For this review, use the dimensioned drawing (mm, ordinates from the lowest corner) and the shaded views. A direction names the side the tool comes from. Round coordinates to 2 decimals unless told otherwise and drop trailing zeros. Write each loop counter-clockwise with the first axis right and the second up, starting at its lowest first coordinate (ties: lowest second). Pieces come first, ordered by that corner, then holes. Notation, with made-up numbers: (-23, -15) - (-7, -15) arc R28 cw to (-7, 19) - close; hole circle Ø1 at (11.25, -30). An arc over 180 degrees is marked (long way). Write each question's results on one line, items separated by ' | '.
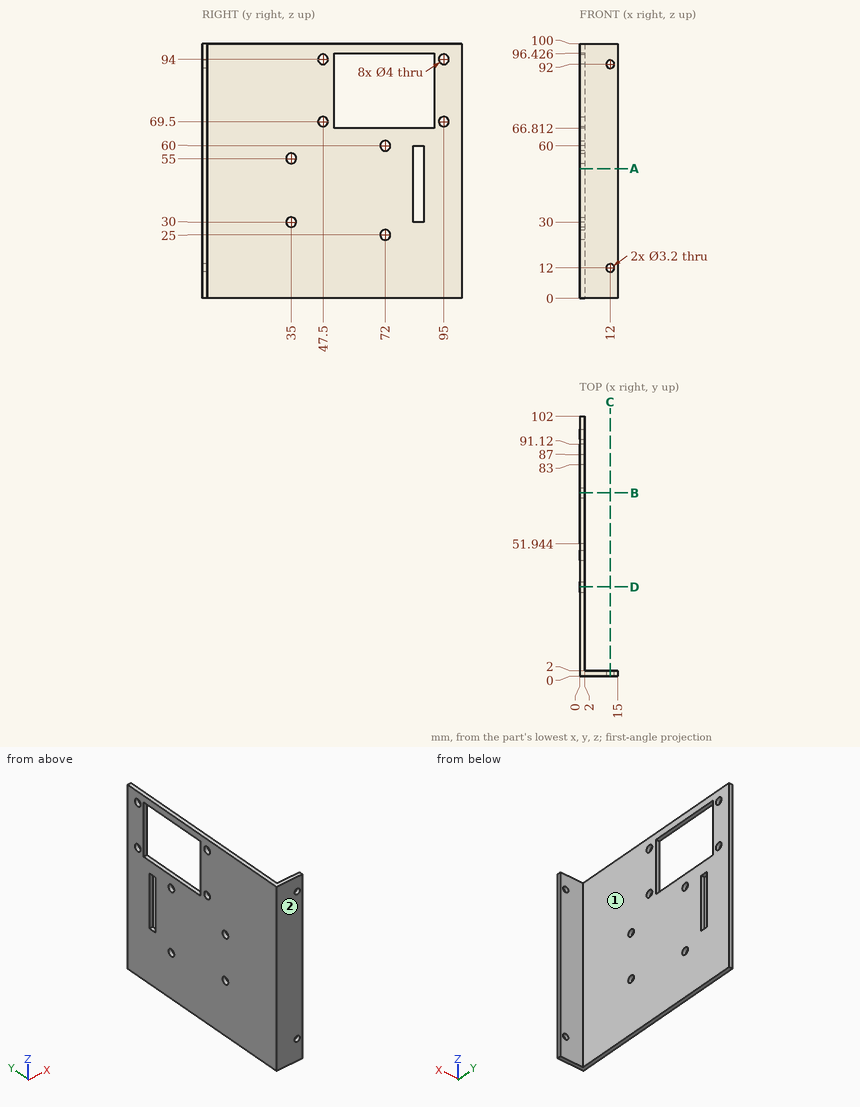
Q1. We need section C-C (x = 12). State the section outline as (y, z) points, plus the area to 3 significant figures.
Evaluation:
outline: (0, 0) - (2, 0) - (2, 10.4) - (0, 10.4) - close; (0, 13.6) - (2, 13.6) - (2, 90.4) - (0, 90.4) - close; (0, 93.6) - (2, 93.6) - (2, 100) - (0, 100) - close | area: 187 mm^2
Q2. We need section A-A (z = 51). State the section outline as (x, y) points.
Evaluation:
outline: (0, 0) - (15, 0) - (15, 2) - (2, 2) - (2, 83) - (0, 83) - close; (0, 87) - (2, 87) - (2, 102) - (0, 102) - close
Q3. We need section B-B (y = 72). State the section outline as (x, z) points (1 decimal).
Evaluation:
outline: (0, 0) - (2, 0) - (2, 23) - (0, 23) - close; (0, 27) - (2, 27) - (2, 58) - (0, 58) - close; (0, 62) - (2, 62) - (2, 66.8) - (0, 66.8) - close; (0, 96.4) - (2, 96.4) - (2, 100) - (0, 100) - close
Q4. Tool access review of the marked faces 1 and 2: name each direction out of +Z, -Z, +X, -X, +Y, -Y from which nothing blocks a thin tool from reaching the whole face with its end or side.
Evaluation:
face 1: +Z, -Z, +X, +Y | face 2: +Z, -Z, +X, -X, -Y
Q5. Insertion check: P1, Ø4, axis at x = 12, z = 92, coming from the -Y side; P2, Ø3.5, axis at y = 72, z = 60, coming from the -X side; P3, Ø1, axis at x = 8.5, z = 39.5, coming from the +Y side; P4, Ø5, axis at y = 72, z = 25, coming from the +X side. Each pin has a flat end and moves straight along its axis. Give the tip position at first contact, or say it passes through.
Evaluation:
P1: stops at y = 0 | P2: passes through | P3: stops at y = 2 | P4: stops at x = 2
Q6. For probe 1 along Y at (x, z) = (1.05, 94) (1 decimal); probe 2 along Z at (x, y) = (12, 0.75); probe 3 along Y at (x, z) = (1.25, 88.5) (1 decimal), list the stretches that pass through material, from the lowest coordinate up.
Evaluation:
probe 1: y = 0 to 45.5, 49.5 to 51.9, 91.1 to 93, 97 to 102 | probe 2: z = 0 to 10.4, 13.6 to 90.4, 93.6 to 100 | probe 3: y = 0 to 51.9, 91.1 to 102
Q7. We need section D-D (y = 35). State the section outline as (x, z) points.
Evaluation:
outline: (0, 0) - (2, 0) - (2, 28) - (0, 28) - close; (0, 32) - (2, 32) - (2, 53) - (0, 53) - close; (0, 57) - (2, 57) - (2, 100) - (0, 100) - close
